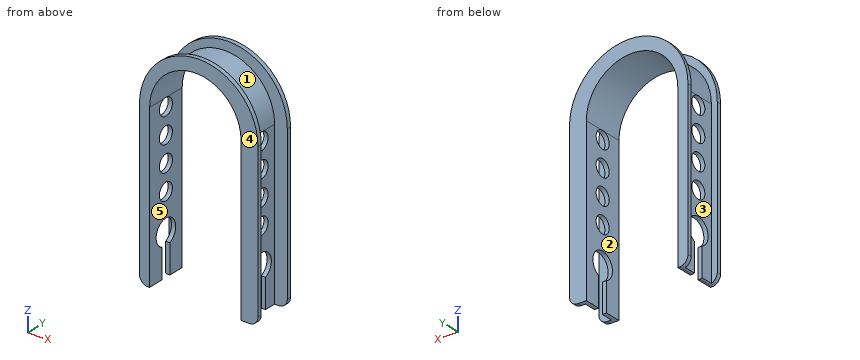
```python
from build123d import *

# Parameters (mm, degrees)
F1_DEPTH  = 50
F2_T      = 5
F4_R      = 10
F5_DEPTH  = 125.1874270275
F6_DEPTH  = 125.1874270275
F7_W      = 40
F7_H      = 10
F8_DEPTH  = 15
F9_W      = 40
F9_H      = 10
F10_DEPTH = 7
F11_W     = 12
F11_H     = 5
F12_DEPTH = 125.1874270275


# Not quite as in the source:
# - a shell that OpenCascade refuses in one call is made with other operations: the cavity is built on its own and cut out
# - a feature names something its author has since deleted; it is built from what else it names


with BuildPart() as f1:
    # F0 (on Front) → F1 (new body)
    with BuildSketch(Plane.XZ):
        with BuildLine():
            Line((-68.1080648237, 65.760188823), (-68.1080648237, -115.239811177))
            ThreePointArc((-68.1080648237, -115.239811177), (-65.1791326356, -122.3108789889), (-58.1080648237, -125.239811177))
            Line((-58.1080648237, -125.239811177), (-56.1080648237, -125.239811177))
            Line((-56.1080648237, -125.239811177), (-56.1080648237, 65.760188823))
            ThreePointArc((-56.1080648237, 65.760188823), (-2.01485131, 119.8534023367), (52.0783622037, 65.760188823))
            Line((52.0783622037, 65.760188823), (52.0783622037, -125.239811177))
            Line((52.0783622037, -125.239811177), (62.0783622037, -125.239811177))
            ThreePointArc((62.0783622037, -125.239811177), (69.1494300156, -122.3108789889), (72.0783622037, -115.239811177))
            Line((72.0783622037, -115.239811177), (72.0783622037, 65.760188823))
            ThreePointArc((72.0783622037, 65.760188823), (1.98514869, 135.8534023367), (-68.1080648237, 65.760188823))
        make_face()
    extrude(amount=F1_DEPTH)

    # F2: shell of thickness 5, made by hand


with BuildPart() as f2_core1:
    # F2_t2: copy of F1
    add(f1.part)

    # the walls: a layer under each face that stays
    f2_faces = [f2_core1.faces().sort_by_distance(p)[0] for p in [
        (52.0783622037, -25, -29.739811177),
        (57.0783622037, -25, -125.239811177),
        (69.1494300156, -25, -122.3108789889),
        (-65.1791326356, -25, -122.3108789889),
        (-57.1080648237, -25, -125.239811177),
        (-56.1080648237, -25, -29.739811177),
        (-2.01485131, -25, 119.8534023367),
        (48.7139576992, 0, 92.3378667511),
        (48.7139576992, -50, 92.3378667511),
    ]]
    thicken(f2_faces, amount=-F2_T, mode=Mode.SUBTRACT)


with BuildPart() as f1_1:
    add(f1.part)

    # what is left inside the walls is the cavity
    f2_cavity = [f2_core1.part.solids().sort_by_distance(p)[0] for p in [
        (1.985149, -31.666667, 135.803402),
    ]]
    add(f2_cavity, mode=Mode.SUBTRACT)

    # F4 (on face) → F5 (cut, through all)
    with BuildSketch(Plane.YZ.offset(57.0783622037)):
        with Locations((-25, 55.9842178226)):
            Circle(F4_R)
        with Locations((-25, 25.9842178226)):
            Circle(F4_R)
        with Locations((-25, -4.0157821774)):
            Circle(F4_R)
        with Locations((-25, -34.0157821774)):
            Circle(F4_R)
    extrude(amount=-F5_DEPTH, mode=Mode.SUBTRACT)

    # F3 (on face) → F6 (cut, through all)
    with BuildSketch(Plane.YZ.offset(57.0783622037)):
        with BuildLine():
            Line((-19, -120.239811177), (-19, -90.9199170358))
            ThreePointArc((-19, -90.9199170358), (-25, -62.1721899509), (-31, -90.9199170358))
            Line((-31, -90.9199170358), (-31, -120.239811177))
            Line((-31, -120.239811177), (-19, -120.239811177))
        make_face()
    extrude(amount=-F6_DEPTH, mode=Mode.SUBTRACT)

    # F7 (on face) → F8 (cut)
    with BuildSketch(Plane.YZ.offset(72.0783622037)):
        with Locations((-25, -120.239811177)):
            Rectangle(F7_W, F7_H)
    extrude(amount=-F8_DEPTH, mode=Mode.SUBTRACT)

    # F9 (on face) → F10 (cut)
    with BuildSketch(Plane(origin=(-68.1080648237, 0, 0), x_dir=(0, -1, 0), z_dir=(-1, 0, 0))):
        with Locations((25, -120.239811177)):
            Rectangle(F9_W, F9_H)
    extrude(amount=-F10_DEPTH, mode=Mode.SUBTRACT)

    # F11 (on face) → F12 (cut, through all)
    with BuildSketch(Plane.YZ.offset(57.0783622037)):
        with Locations((-25, -122.739811177)):
            Rectangle(F11_W, F11_H)
    extrude(amount=-F12_DEPTH, mode=Mode.SUBTRACT)


solid = f1_1.part
```
Model file for the job. Use its own axes, mm. Face numbers are marked on the shaded views. A direction names the side the tool comes from. Coordinates: 2 decimals unless noted, no trailing zeros. Order: outer loops, then holes, each group sorted by start corner. A loop starts at its lowest first (then second) coordinate and runs counter-clockwise, first axis right, second up. Notation, with made-up numbers: (12, -20.5) - (58, -20.5) arc R22 ccw to (58, 8.5) - close; hole circle Ø10 at (83, 4). An arc over 180 degrees is marked (long way). Return JSON: item names as keys, results as strings. Group by question number.
1) Saw through at B-B, the plane z = 59. Write the cut outline in (x, y).
2) Probe line 1 (X direction, y = -16.5, z = -21); line 2 (X direction, y = -3, z = 24); line 3 (Y direction, x = 65.5, z = -73.5). List the from-to ranges inside material, lowest first. Write a range as from..to.
3) Tool access for the marked faces 4 and 5: list every direction of +Z, -Z, +X, -X, +Y, -Y with a clear straight run to the whole face (end or side of a thin tool).
4) Saw through at C-C, the plane x = -37. Write the cut outline in (y, z).
5) Saw through at D-D, the plane z = 19. Write the cut outline in (x, y).
6) Saw through at A-A, the plane z = 86. Write the cut outline in (x, y).
7) Mould opens along X. For the marked faces 1, 2 and 3 say: released by +X, released by -X, zero draft, split by the parting line, or undercut.
8) Flat gauge pins, fed straight in: P1, Ø4, axis at y = -42.5, z = -4.5, coming from the +X side; P2, Ø1, axis at y = -39, z = 80.5, coming from the -X side; P3, Ø10, axis at x = 51, z = -31, coming from the -Y side; P4, Ø1, axis at y = -12, z = -40.5, coming from the -X side. Where does each tip first touch, or does it go through?
Values found:
{
 "1": {"outline": "(-68.11, -50) - (-56.11, -50) - (-56.11, -34.53) - (-61.11, -34.53) - (-61.11, -45) - (-68.11, -45) - close; (-68.11, -5) - (-61.11, -5) - (-61.11, -15.47) - (-56.11, -15.47) - (-56.11, 0) - (-68.11, 0) - close; (52.08, -50) - (72.08, -50) - (72.08, -45) - (57.08, -45) - (57.08, -34.53) - (52.08, -34.53) - close; (52.08, -15.47) - (57.08, -15.47) - (57.08, -5) - (72.08, -5) - (72.08, 0) - (52.08, 0) - close"},
 "2": {"line 1": "x = -61.11..-56.11, 52.08..57.08", "line 2": "x = -68.11..-56.11, 52.08..72.08", "line 3": "y = -50..-45, -5..0"},
 "3": {"face 4": "+Z, -Z, +X, -X, -Y", "face 5": "-Z, +Y, -Y"},
 "4": {"outline": "(-50, 107.02) - (0, 107.02) - (0, 124.01) - (-5, 124.01) - (-5, 113.38) - (-45, 113.38) - (-45, 124.01) - (-50, 124.01) - close"},
 "5": {"outline": "(-68.11, -50) - (-56.11, -50) - (-56.11, -32.16) - (-61.11, -32.16) - (-61.11, -45) - (-68.11, -45) - close; (-68.11, -5) - (-61.11, -5) - (-61.11, -17.84) - (-56.11, -17.84) - (-56.11, 0) - (-68.11, 0) - close; (52.08, -50) - (72.08, -50) - (72.08, -45) - (57.08, -45) - (57.08, -32.16) - (52.08, -32.16) - close; (52.08, -17.84) - (57.08, -17.84) - (57.08, -5) - (72.08, -5) - (72.08, 0) - (52.08, 0) - close"},
 "6": {"outline": "(-65.12, -50) - (-52.18, -50) - (-52.18, 0) - (-65.12, 0) - (-65.12, -5) - (-57.53, -5) - (-57.53, -45) - (-65.12, -45) - close; (48.15, -50) - (69.09, -50) - (69.09, -45) - (53.5, -45) - (53.5, -5) - (69.09, -5) - (69.09, 0) - (48.15, 0) - close"},
 "7": {"face 1": "split by the parting line", "face 2": "undercut", "face 3": "released by -X"},
 "8": {"P1": "stops at x = 57.08", "P2": "stops at x = -59.37", "P3": "stops at y = -50", "P4": "stops at x = -61.11"}
}
